Can you work these out from the drawing? Everything is in mm from the part's minimum corner. A direction names the side the tool comes from. Round coordinates to 2 decimals unless told otherwise and drop trailing zeros. Order: outer loops, then holes, each group sorted by start corner. A loop starts at its lowest first (then second) coordinate and runs counter-clockwise, first axis right, second up. Notation, with made-up numbers: M 46,36.5 L 104,36.5 A21 ccw 104,72.5 Z; hole C 79.25,72.25 d7. An arc over 180 degrees is marked long. Write item = value, one per line. Start each with the question number.
Item 1: We'd pull the mould along Y, two halves only. Please class the marked faces 4, 5, 6 and 7: pulls with the +Y half, pulls with the -Y half, needs draft (parallel to the pull), parting line crosses it, or undercut.
Item 2: I want a section at C-C, the plane z = 5.25. List the corners of the cut face in (x, y) for me.
Item 3: For the marked faces 1, 2 and 3, which set-ups out of +Z, -Z, +X, -X, +Y, -Y let a thin tool reach every point of the face, with its end or its side?
Item 4: Please list where these lines run through material, in increasing order: L1, parallel to Y at x = 8.75, z = 4.6; L2, parallel to X at y = 7.5, z = 5.2; L3, parallel to Y at x = 4, z = 1.8.
Item 5: I'm going to push flat-ended pins straight in: P1, Ø5, axis at x = 2.5, y = 30, coming from the +Z side; P2, Ø3, axis at y = 34.5, z = 1.5, coming from the +X side; P3, Ø1.8, axis at x = 16, z = 4, coming from the -Y side; P4, Ø1.8, axis at y = 38, z = 4, coming from the -X side. Where does each tip first touch, or does it pass through?
Item 6: I want a section at A-A, the plane y = 11. List the corners of the cut face in (x, z) for me.
Item 7: I want a section at B-B, the plane x = 10.5. List the corners of the cut face in (y, z) for me, plus the area to 3 significant figures.
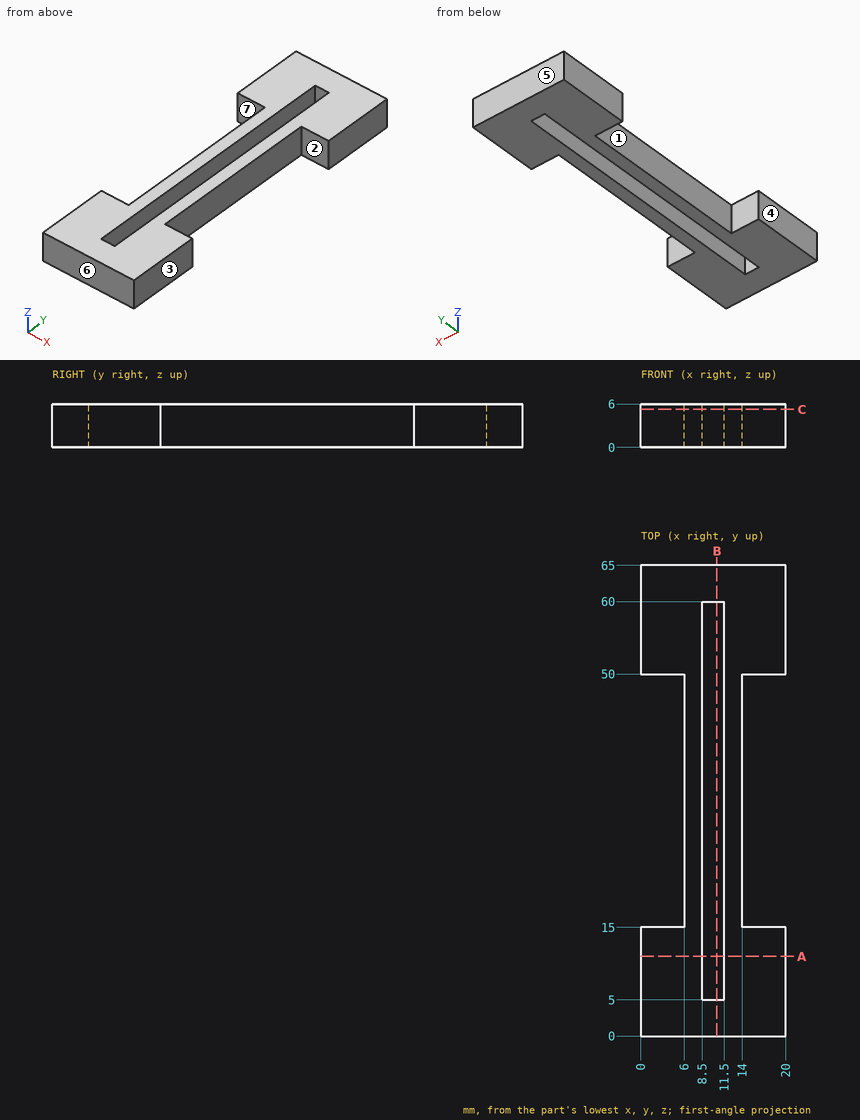
Filled in:
q1.face_4 = needs draft
q1.face_5 = pulls with the +Y half
q1.face_6 = pulls with the -Y half
q1.face_7 = undercut
q2.outline = M 0,0 L 20,0 L 20,15 L 14,15 L 14,50 L 20,50 L 20,65 L 0,65 L 0,50 L 6,50 L 6,15 L 0,15 Z; hole M 8.5,5 L 11.5,5 L 11.5,60 L 8.5,60 Z
q3.face_1 = +Z, -Z, -X
q3.face_2 = +Z, -Z, +X
q3.face_3 = +Z, -Z, +X, +Y, -Y
q4.L1 = 0 to 5, 60 to 65
q4.L2 = 0 to 8.5, 11.5 to 20
q4.L3 = 0 to 15, 50 to 65
q5.P1 = through
q5.P2 = 14
q5.P3 = 0
q5.P4 = 6
q6.outline = M 0,0 L 8.5,0 L 8.5,6 L 0,6 Z; M 11.5,0 L 20,0 L 20,6 L 11.5,6 Z
q7.outline = M 0,0 L 5,0 L 5,6 L 0,6 Z; M 60,0 L 65,0 L 65,6 L 60,6 Z
q7.area = 60.0 mm^2
